Input: part model. Units: mm. Frame: model coordinates. Face numbers are marked on the shaded views. A direction names the side the tool comes from. Give positions to 0.01 mm unless a question says otherwise; leave off trailing zeros. Loops run counter-clockwise (first coordinate to the right, second up) from the corner with the lowest first, then second, coordinate; pieces in that order, holes last. Notation, with made-up numbers: (12.5, 44) - (51.5, 44) arc R18 cw to (51.5, 64) - close; hole circle Ø4 at (64, -32.75). An arc over 180 degrees is marked (long way). Answer as a JSON object with one key per item and string values. Group by question number.
(1) Section query D-D (x = 17). Return loops of the section in (y, z), plus the area to 3 significant figures.
(2) Mould query, pull axis Y, two halves, no side actions, for the marked faces 5, 6 and 7. Classes: +Y half, -Y half, draft (parallel to the pull), parting line (faces both ways), or undercut.
(3) Material intervals for L1, parallel to Y at x = 64.5, z = 4.5; L2, parallel to Y at x = 2.5, z = 25; L3, parallel to Z at x = 45, y = -36, sorted ascending.
(4) Pin query (flat end, axial travel): P1, Ø10, axis at y = -18.5, z = 33, coming from the +X side; P2, Ø1.5, axis at x = 59.5, z = 12, coming from the -Y side; P3, Ø13.5, axis at x = 43.5, y = -18.5, coming from the +Z side; P4, Ø12, axis at y = -9.5, z = 10.5, coming from the -X side. Return the tip coordinate at first contact, or that it passes through.
(5) Section query A-A (x = 55). Return loops of the section in (y, z), plus the area to 3 significant figures.
(6) Section query B-B (y = -9). Return loops of the section in (x, z).
(7) Access query for the marked faces 1, 2, 3 and 4. Directions: +Z, -Z, +X, -X, +Y, -Y. A direction counts if a zero-diameter tool reaches every point of the face in a straight line with its end or side. Return the directions, or none.
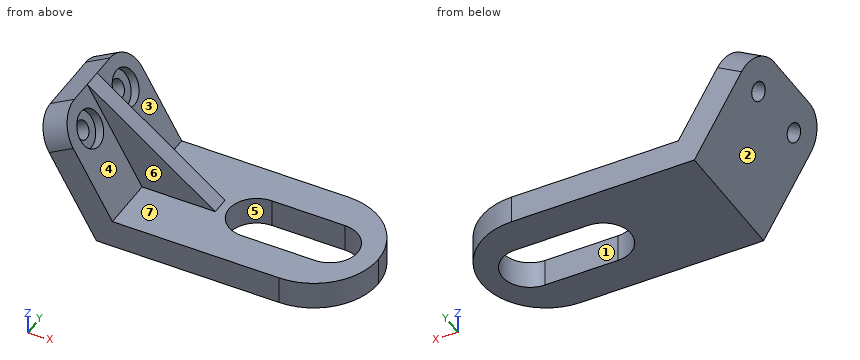
```python
from build123d import *

# Parameters (mm, degrees)
F1_DEPTH  = 44.704
F3_R      = 22.35199
F5_R      = 10.922
F4_R      = 3.175
F6_DEPTH  = 28.5637839421
F4_R_2    = 6.35
F7_DEPTH  = 3.175
F8_DEPTH  = 9.653
F11_DEPTH = 3.175


# Not quite as in the source:
# - a fillet or chamfer is up to 0.001 mm smaller than in the source, because OpenCascade refuses the exact size


with BuildPart() as f1:
    # F0 (on Front) → F1 (new body)
    with BuildSketch(Plane.XZ):
        Polygon((-21.8362923991, 37.8215678842), (0, 0), (85.852, 0), (85.852, 9.652), (30.9725847982, 9.652), (5.5725847982, 9.652), (-13.4774152018, 42.6475678842), align=None)
    extrude(amount=F1_DEPTH)

    # F3 (radius 22.352 in the source; OpenCascade refuses exactly that, so slightly less here)
    f3_edges = [f1.edges().sort_by_distance(p)[0] for p in [
        (85.852, -44.704, 4.826),
        (85.852, 0, 4.826),
    ]]
    fillet(f3_edges, radius=F3_R)

    # F5
    f5_edges = [f1.edges().sort_by_distance(p)[0] for p in [
        (-17.656854, -44.704, 40.234568),
        (-17.656854, 0, 40.234568),
    ]]
    fillet(f5_edges, radius=F5_R)

    # F4 (on face) → F6 (cut, through all)
    with BuildSketch(Plane(origin=(8.3588771973, 0, 4.826), x_dir=(0, 1, 0), z_dir=(0.8660254038, 0, 0.5))):
        with Locations((-33.782, 32.7505847982)):
            Circle(F4_R)
        with Locations((-10.922, 32.7505847982)):
            Circle(F4_R)
    extrude(amount=-F6_DEPTH, mode=Mode.SUBTRACT)

    # F4 (on face) → F7 (cut)
    with BuildSketch(Plane(origin=(8.3588771973, 0, 4.826), x_dir=(0, 1, 0), z_dir=(0.8660254038, 0, 0.5))):
        with Locations((-33.782, 32.7505847982)):
            Circle(F4_R_2)
        with Locations((-33.782, 32.7505847982)):
            Circle(F4_R, mode=Mode.SUBTRACT)
        with Locations((-10.922, 32.7505847982)):
            Circle(F4_R_2)
        with Locations((-10.922, 32.7505847982)):
            Circle(F4_R, mode=Mode.SUBTRACT)
    extrude(amount=-F7_DEPTH, mode=Mode.SUBTRACT)

    # F2 (on face) → F8 (cut, through all)
    with BuildSketch(Plane.XY.offset(9.652)):
        with BuildLine():
            Line((43.6725847982, -32.004), (69.0725847982, -32.004))
            ThreePointArc((69.0725847982, -32.004), (78.7245847982, -22.352), (69.0725847982, -12.7))
            Line((69.0725847982, -12.7), (43.6725847982, -12.7))
            ThreePointArc((43.6725847982, -12.7), (34.0205847982, -22.352), (43.6725847982, -32.004))
        make_face()
    extrude(amount=-F8_DEPTH, mode=Mode.SUBTRACT)

    # F10 (on offset) → F11 (join, symmetric)
    with BuildSketch(Plane.XZ.offset(22.352)):
        Polygon((30.9725847982, 9.652), (-13.4774152018, 42.6475678842), (-8.0164152018, 33.1888384241), (5.5725847982, 9.652), align=None)
    extrude(amount=F11_DEPTH, both=True)


solid = f1.part
```
Recorded:
{
 "1": {"outline": "(-44.7, 0) - (0, 0) - (0, 9.65) - (-19.18, 9.65) - (-19.18, 20.02) - (-25.53, 20.02) - (-25.53, 9.65) - (-44.7, 9.65) - close", "area": "497 mm^2"},
 "2": {"face 5": "undercut", "face 6": "-Y half", "face 7": "draft"},
 "3": {"L1": "y = -44.68 to -32, -12.7 to -0.02", "L2": "y = -25.53 to -19.18", "L3": "z = 0 to 9.65"},
 "4": {"P1": "stops at x = 6.19", "P2": "passes through", "P3": "stops at z = 9.65", "P4": "stops at x = -9.53"},
 "5": {"outline": "(-44.7, 0) - (-32, 0) - (-32, 9.65) - (-44.7, 9.65) - close; (-12.7, 0) - (0, 0) - (0, 9.65) - (-12.7, 9.65) - close", "area": "245 mm^2"},
 "6": {"outline": "(-21.75, 37.67) - (-17.64, 30.55) - (-12.03, 33.79) - (-13.79, 36.84) - (-11.04, 38.43) - (-13.39, 42.5) - close; (-15.11, 26.17) - (0, 0) - (81.43, 0) - (81.43, 9.65) - (5.57, 9.65) - (-4.99, 27.95) - (-7.74, 26.36) - (-9.5, 29.41) - close"},
 "7": {"face 1": "+Z, -Z", "face 2": "-Z, -X, +Y, -Y", "face 3": "+Z, +X, +Y", "face 4": "+Z, +X, -Y"}
}
